Could you check a few things on this drawing? It's one solid part, dimensions in mm from its lowest x, y, z. A direction names the side the tool comes from. Round coordinates to 2 decimals unless told otherwise and drop trailing zeros. Loops run counter-clockwise (first coordinate to the right, second up) from the corner with the lowest first, then second, coordinate; pieces in that order, holes last. Notation, with made-up numbers: (8.25, -23) -> (42.25, -23) arc R23 ccw to (42.25, -11) -> close; hole circle Ø9 at (33.5, 3.25). An arc over 180 degrees is marked (long way). Put each result on its own line as item: value. Start each with the question number.
1. Imagine slicing it at A-A, the plane x = 9. Please give me the cut outline in (y, z).
2. I need wall thicknesses on line 1 (Y direction, x = 19, z = 56); line 2 (X direction, y = 9, z = 8); line 3 (X direction, y = 5, z = 38.5). Which ranges of each line are inside material? Lowest first, please. Write a range as [from, to].
3. Imagine slicing it at B-B, the plane y = 52. Please give me the cut outline in (x, z), and give its area (3 significant figures).
4. If we mould it in two halves opening along X, with no side actions, what happens to the marked faces 1, 2 and 3? For each: pulls with the +X half, pulls with the -X half, needs draft (parallel to the pull), parting line crosses it, or undercut.
5. Which directions (+Z, -Z, +X, -X, +Y, -Y) give clear straight access to the entire face, cutting with the end or side of a thin tool? Please do the marked faces 4 and 5.
6. Imagine slicing it at C-C, the plane z = 39.5. Please give me the cut outline in (x, y).
7. I'm going to push flat-ended pins straight in: P1, Ø10, axis at x = 18.5, y = 20, coming from the -Z side; P2, Ø3, axis at x = 4, z = 46.5, coming from the -Y side. Where does each tip first touch, or does it pass through?
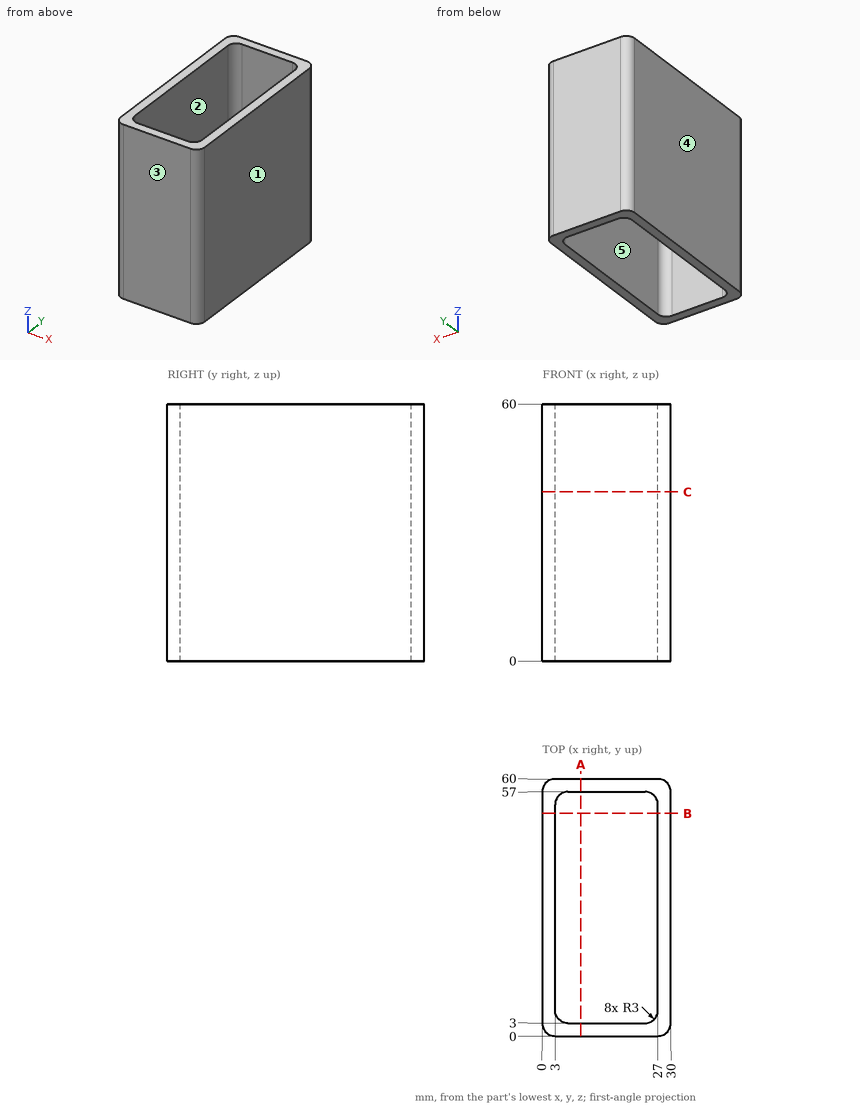
Entries:
1. outline: (0, 0) -> (3, 0) -> (3, 60) -> (0, 60) -> close; (57, 0) -> (60, 0) -> (60, 60) -> (57, 60) -> close
2. line 1: [0, 3], [57, 60]
2. line 2: [0, 3], [27, 30]
2. line 3: [0, 3.17], [26.83, 30]
3. outline: (0, 0) -> (3, 0) -> (3, 60) -> (0, 60) -> close; (27, 0) -> (30, 0) -> (30, 60) -> (27, 60) -> close
3. area: 360 mm^2
4. face 1: pulls with the +X half
4. face 2: undercut
4. face 3: needs draft
5. face 4: +Z, -Z, -X, +Y, -Y
5. face 5: +Z, -Z
6. outline: (0, 3) arc R3 ccw to (3, 0) -> (27, 0) arc R3 ccw to (30, 3) -> (30, 57) arc R3 ccw to (27, 60) -> (3, 60) arc R3 ccw to (0, 57) -> close; hole (3, 6) arc R3 ccw to (6, 3) -> (24, 3) arc R3 ccw to (27, 6) -> (27, 54) arc R3 ccw to (24, 57) -> (6, 57) arc R3 ccw to (3, 54) -> close
7. P1: through
7. P2: y = 0
